```python
from build123d import *

# Parameters (mm, degrees)
F6_ANGLE = 270
F7_T     = -2


with BuildPart() as f6:
    # F5 (on Right) → F6 (revolve)
    with BuildSketch(Plane.YZ):
        Polygon((0, 0), (28.5, 0), (28.5, 35), (16, 52), (16, 107), (27.5, 122), (27.5, 159), (0, 159), align=None)
    revolve(axis=Axis((0, 0, 79.5), (0, 0, 1)), revolution_arc=F6_ANGLE)

    # F7
    f7_openings = [f6.faces().sort_by_distance(p)[0] for p in [
        (0, 12.000093, 78.927374),
        (-3.890454, -3.890454, 159),
        (12.000093, 0, 78.927374),
        (-4.031925, -4.031925, 0),
    ]]
    offset(amount=F7_T, openings=f7_openings, kind=Kind.INTERSECTION)


solid = f6.part
```
CAD build for the part. Positions are in the model's coordinates, mm. A direction names the side the tool comes from. Coordinates: 2 decimals unless noted, no trailing zeros. Order: outer loops, then holes, each group sorted by start corner. A loop starts at its lowest first (then second) coordinate and runs counter-clockwise, first axis right, second up. Notation, with made-up numbers: (57.25, -14.5) - (72.25, -14.5) arc R8 cw to (72.25, -9.5) - close; hole circle Ø1 at (64.25, -29.5). An arc over 180 degrees is marked (long way). Use a Markdown table: item, result. Add a question column.
(1) Pull direction X, two halves, no side cores. Call faces 1 (the face through (0, 15.8, 79.9)), 2 (the face through (15.8, 0, 79.9)), 3 (the face through (-19.346, -18.11, 17.412)), 4 (the face through (-18.616, -17.427, 141.093)): +X half, -X half, draft (parallel to the pull), parting line (faces both ways), or undercut.
(2) Saw through at A-A (z = 113). Give the cut face in (x, y).
(3) Which spindle directions (+Z, -Z, +X, -X, +Y, -Y) get a long thin tool onto all of the face, cutting with end or side? Do faces 5 (the face through (-10.664, -9.982, 50.518)), 6 (the face through (-11.681, -10.934, 79.885)), 7 (the face through (-20.08, -18.79, 140.76)). Say none if no direction does.
(4) Drill centre lines: line 1 along Z through (x, y) = (-2.5, -17); line 2 along Z through (x, y) = (25.5, -5.5); line 3 along Y through (x, z) = (-19, 133.5). Where is each one in solid material? Low to high. Write a range as [from, to].
(5) Flat gauge pins, fed straight in: pin 1 (3 mm diameter, centred on x = 3.5, z = 127.5, fed in from -Y); pin 2 (1 mm diameter, centred on x = 6.5, z = 75, fed in from -Y); pin 3 (12 mm diameter, centred on y = -12.5, z = 55, fed in from +X); pin 4 (22.5 mm diameter, centred on x = 0, y = 0, fed in from +Z). Where does each tip first touch, or does it go through?
Solved:
| question | item | result |
|---|---|---|
| 1 | face 1 | +X half |
| 1 | face 2 | draft |
| 1 | face 3 | undercut |
| 1 | face 4 | undercut |
| 2 | outline | (0, 18.08) - (0, 20.6) arc R20.6 ccw (long way) to (20.6, 0) - (18.08, 0) arc R18.08 cw (long way) to start |
| 3 | face 5 | -Z |
| 3 | face 6 | none |
| 3 | face 7 | +Z |
| 4 | line 1 | z = [47.02, 50.39], [108.54, 111.83] |
| 4 | line 2 | z = [34.91, 38.28], [120.16, 159] |
| 4 | line 3 | y = [-19.88, -17.01], [17.01, 19.88] |
| 5 | pin 1 | stops at y = -27.43 |
| 5 | pin 2 | stops at y = -14.83 |
| 5 | pin 3 | stops at x = 14.87 |
| 5 | pin 4 | passes through |
